Can you work these out from the drawing? Everything is in mm from the part's minimum corner. Round coordinates to 2 decimals unless told otherwise and drop trailing zeros. Loops run counter-clockwise (first coordinate to the right, second up) from the corner with the lowest first, then second, coordinate; pieces in that order, holes last. Notation, with made-up numbers: (25.25, 16) -> (59.25, 16) arc R27 cw to (59.25, 41) -> close; hole circle Ø3 at (2.5, 57). An arc over 180 degrees is marked (long way). Answer as a JSON object with one key per item and string values.
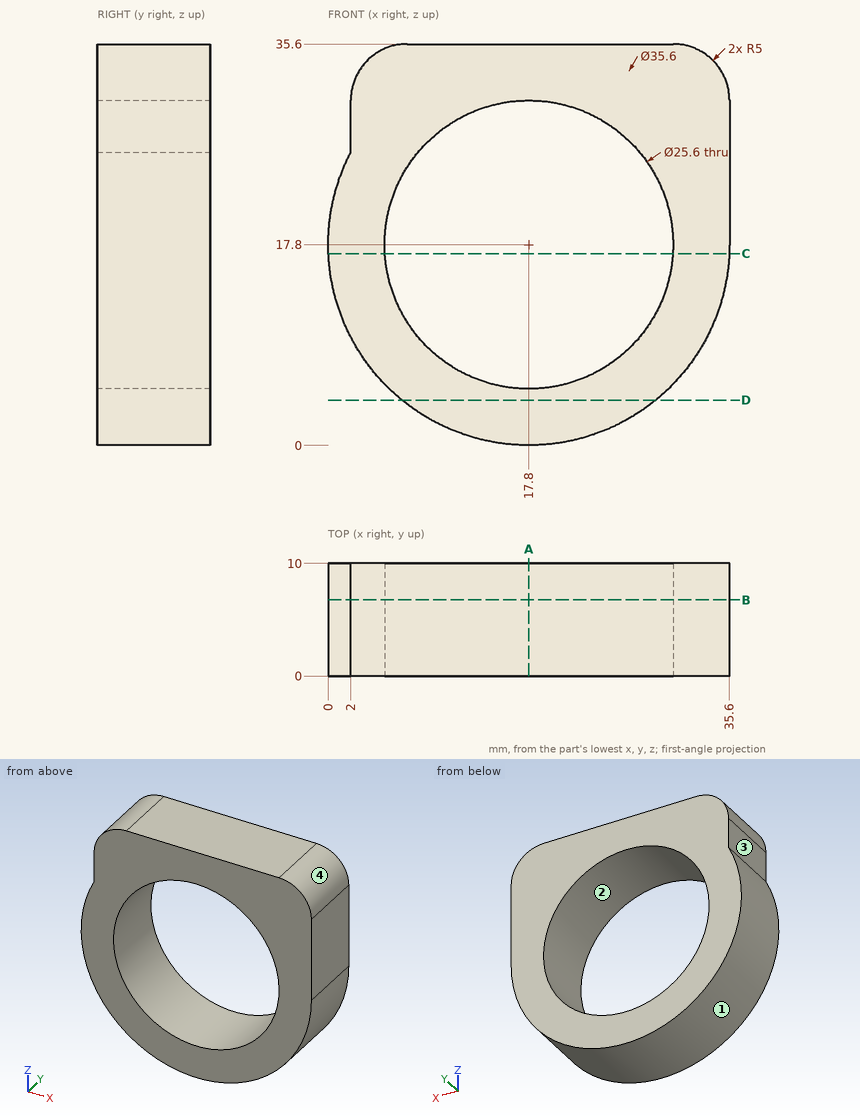
Q1. We'd pull the mould along Z, two halves only. Please class the marked faces 1, 2, 3 and 4: pulls with the +Z half, pulls with the -Z half, needs draft (parallel to the pull), parting line crosses it, or undercut.
Determined:
{"face 1": "parting line crosses it", "face 2": "undercut", "face 3": "needs draft", "face 4": "pulls with the +Z half"}
Q2. I want a section at D-D, the plane z = 4. Write out the boundary of the cut face in (x, y), then the cut area to 3 significant figures.
Determined:
{"outline": "(6.56, 0) -> (29.04, 0) -> (29.04, 10) -> (6.56, 10) -> close", "area": "225 mm²"}
Q3. I'm going to push a flat-ended pin straight in: pin 1 (1.4 mm diameter, centred on y = 3, z = 27, fed in from -X). Where does the tip first touch, or does it pass through?
Determined:
{"pin 1": "x = 2"}
Q4. If I drill on L1, parallel to X at y = 1, z = 18; L2, parallel to Z at x = 11, y = 3.5; L3, parallel to X at y = 8.25, z = 11.5, over which ranges is the centre line in solid material (lowest first)? Write a range as [from, to].
Determined:
{"L1": "[0, 5], [30.6, 35.6]", "L2": "[1.35, 6.96], [28.64, 35.6]", "L3": "[1.15, 6.66], [28.94, 34.45]"}
Q5. I want a section at C-C, the plane z = 17. Write out the boundary of the cut face in (x, y), then the cut area to 3 significant figures.
Determined:
{"outline": "(0.02, 0) -> (5.03, 0) -> (5.03, 10) -> (0.02, 10) -> close; (30.57, 0) -> (35.58, 0) -> (35.58, 10) -> (30.57, 10) -> close", "area": "100 mm²"}
Q6. I want a section at A-A, the plane x = 17.8. Write out the boundary of the cut face in (y, z), then the cut area to 3 significant figures.
Determined:
{"outline": "(0, 0) -> (10, 0) -> (10, 5) -> (0, 5) -> close; (0, 30.6) -> (10, 30.6) -> (10, 35.6) -> (0, 35.6) -> close", "area": "100 mm²"}
Q7. I want a section at B-B, the plane y = 6.75. Write out the boundary of the cut face in (x, z).
Determined:
{"outline": "(2, 26) arc R17.8 ccw (long way) to (35.6, 17.8) -> (35.6, 30.6) arc R5 ccw to (30.6, 35.6) -> (7, 35.6) arc R5 ccw to (2, 30.6) -> close; hole circle Ø25.6 at (17.8, 17.8)"}
